```python
from build123d import *

# Parameters (mm, degrees)
F3_R     = 127
F0_DEPTH = 254
F1_T     = -20.32
F2_R     = 10


with BuildPart() as f0:
    # F3 (on Top) → F0 (new body)
    with BuildSketch(Plane.XY):
        Circle(F3_R)
    extrude(amount=F0_DEPTH)

    # F1
    f1_openings = [f0.faces().sort_by_distance(p)[0] for p in [
        (0, 0, 254),
    ]]
    offset(amount=F1_T, openings=f1_openings)

    # F2
    f2_edges = [f0.edges().sort_by_distance(p)[0] for p in [
        (-106.68, 0, 254),
    ]]
    fillet(f2_edges, radius=F2_R)


solid = f0.part
```
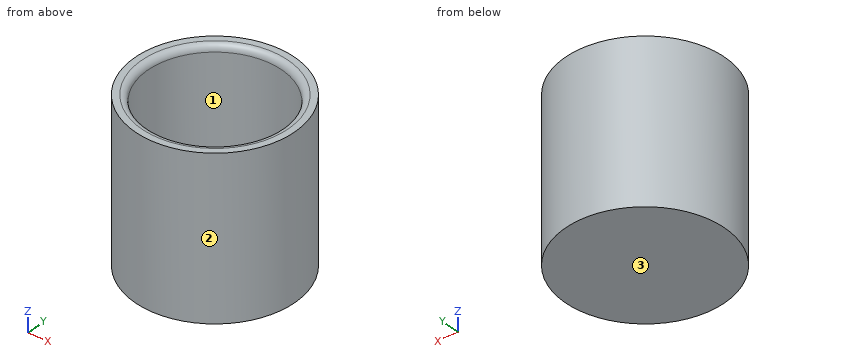
Could you check a few things on this model? Use its own coordinates, in mm. Face numbers are marked on the shaded views. Round coordinates to 2 decimals unless told otherwise and drop trailing zeros. Loops run counter-clockwise (first coordinate to the right, second up) from the corner with the lowest first, then second, coordinate; pieces in that order, holes last. Notation, with made-up numbers: (-36.75, -39.75) -> (-26.75, -39.75) arc R27 cw to (-26.75, -4.75) -> close; hole circle Ø8 at (81, -24.5). An arc over 180 degrees is marked (long way). Put each result on its own line as item: value.
Q1. Thinking about a two-plate mould opening in X: for the marked faces 1, 2 and 3, which applies, pulls with the +X half, pulls with the -X half, needs draft (parallel to the pull), parting line crosses it, or undercut?
Checks:
face 1: undercut
face 2: parting line crosses it
face 3: needs draft
Q2. I want a section at D-D on z = 16. Write out the boundary of the cut face in (x, y), and give its area (3 significant figures).
Checks:
outline: circle Ø254 at (0, 0)
area: 50,700 mm2
Q3. For pin 1 Ø8 at (x, z) = (100, 92) entering from -Y; pin 2 Ø1.5 at (y, z) = (82, 176) entering from -X; pin 3 Ø2 at (x, z) = (-58.5, 225) entering from +Y; pin 4 Ø1.5 at (x, y) = (89, 94) entering from +Z, each with a flat end and sliding along its axis, tell me the tip position at first contact or that it passes through.
Checks:
pin 1: y = -83.14
pin 2: x = -97.61
pin 3: y = 113.24
pin 4: through
Q4. Please list where these lines run through material, in increasing order: line 1 (Y direction, x = 0, z = 86); line 2 (Z direction, x = -47.5, y = 44); line 3 (X direction, y = -10.5, z = 164.5). Write a range as from..to.
Checks:
line 1: -127..-106.68, 106.68..127
line 2: 0..20.32
line 3: -126.57..-106.16, 106.16..126.57
Q5. I want a section at A-A on y = 0. Write out the boundary of the cut face in (x, z).
Checks:
outline: (-127, 0) -> (127, 0) -> (127, 254) -> (116.68, 254) arc R10 ccw to (106.68, 244) -> (106.68, 20.32) -> (-106.68, 20.32) -> (-106.68, 244) arc R10 ccw to (-116.68, 254) -> (-127, 254) -> close
Q6. I want a section at B-B on z = 188. Write out the boundary of the cut face in (x, y).
Checks:
outline: circle Ø254 at (0, 0); hole circle Ø213.36 at (0, 0)
